from build123d import *

# Parameters (mm, degrees)
SKETCH1_R               = 5
BOSS_EXTRUDE1_DEPTH     = 35
SKETCH1_3_R             = 8
SKETCH1_3_R_2           = 5
BOSS_EXTRUDE2_DEPTH     = 2
SKETCH3_R               = 1
CUT_EXTRUDE3_DEPTH      = 9
CUT_EXTRUDE3_DEPTH_BACK = 9
FILLET1_R               = 0.5


with BuildPart() as part:
    # Sketch1 → Boss-Extrude1 (new body)
    with BuildSketch(Plane.XY):
        Circle(SKETCH1_R)
    extrude(amount=BOSS_EXTRUDE1_DEPTH)

    # Sketch1<3> → Boss-Extrude2 (add)
    with BuildSketch(Plane.XY):
        Circle(SKETCH1_3_R)
        Circle(SKETCH1_3_R_2, mode=Mode.SUBTRACT)
    extrude(amount=BOSS_EXTRUDE2_DEPTH)

    # Sketch3 → Cut-Extrude3 (cut, two sides)
    with BuildSketch(Plane(origin=(0, 0, 0), x_dir=(0, 0, -1), z_dir=(1, 0, 0))) as cut_extrude3_sk:
        with Locations((-30, 0)):
            Circle(SKETCH3_R)
    extrude(amount=CUT_EXTRUDE3_DEPTH, mode=Mode.SUBTRACT)
    extrude(cut_extrude3_sk.sketch, amount=-CUT_EXTRUDE3_DEPTH_BACK, mode=Mode.SUBTRACT)

    # Fillet1
    fillet1_edges = [part.edges().sort_by_distance(p)[0] for p in [
        (-5, 0, 35),
    ]]
    fillet(fillet1_edges, radius=FILLET1_R)


solid = part.part
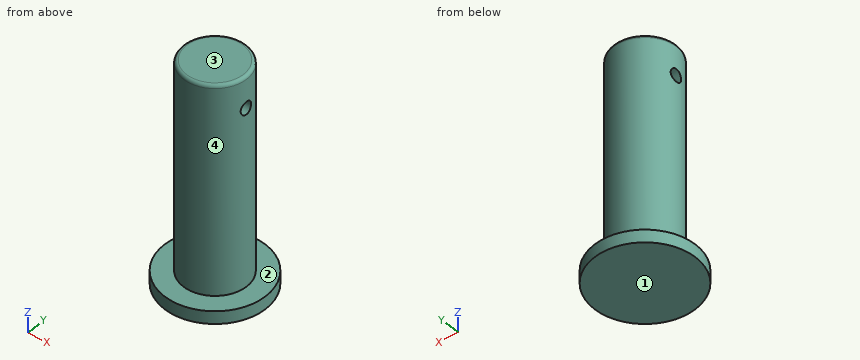
Work out the finished part from the listing and answer in its coordinate system (mm). Face numbers are marked on the shaded views. A direction names the side the tool comes from. Give positions to 0.01 mm unless a question says otherwise; leave off trailing zeros. Order: outer loops, then holes, each group sorted by start corner. A loop starts at its lowest first (then second) coordinate and runs counter-clockwise, first axis right, second up. Notation, with made-up numbers: (23, 89.25) - (52, 89.25) arc R26 ccw to (52, 110.25) - close; hole circle Ø3 at (87.25, 22.25). An arc over 180 degrees is marked (long way). Answer as CSV lines item,"result". Start each with the question number.
Q1. The part is cut by section D-D (x = 6.75). Write down the section's boundary in (y, z).
Q2. The part is cut by section C-C (z = 30). Write down the section's boundary in (x, y), then the cut area to 3 significant figures.
Q3. The part is cut by section A-A (y = 0). Write down the section's boundary in (x, z).
Q4. Given pin 1 Ø5 at (x, y) = (-4.5, -1) entering from +Z; pin 2 Ø3 at (y, z) = (0, 30) entering from -X; pin 3 Ø6 at (x, z) = (-5, 20.5) entering from -Y; pin 4 Ø8 at (x, z) = (5.5, 21) entering from -Y, each flat-ended and moving along its own axis, determine where each tip first touches the part or whether it passes through.
Q5. The mould has two halves that part along X. Classify the marked faces 3 and 4: +X half, -X half, draft (parallel to the pull), parting line (faces both ways), or undercut.
Q6. Find the intervals of material crossed by L1, parallel to Z at x = 2.05, y = 0; L2, parallel to Z at x = -0.75, y = 7.25; L3, parallel to Y at x = -3.15, z = 30, in increasing order. Write a range as [from, to].
Q7. The part is cut by section B-B (z = 17). Write down the section's boundary in (x, y).
Q8. For the marked faces 1 and 2, determine the directions among +Z, -Z, +X, -X, +Y, -Y from which every point of the face is accessible in a straight line to the end or side of a thin tool.
Check result:
1,outline,"(-4.29, 0) - (4.29, 0) - (4.29, 2) - (-4.29, 2) - close"
2,outline,"(-4.9, -1) arc R5 ccw to (4.9, -1) - close; (-4.9, 1) - (4.9, 1) arc R5 ccw to start"
2,area,"58.7 mm²"
3,outline,"(-8, 0) - (8, 0) - (8, 2) - (5, 2) - (5, 29) - (-5, 29) - (-5, 2) - (-8, 2) - close; (-5, 31) - (5, 31) - (5, 34.5) arc R0.5 ccw to (4.5, 35) - (-4.5, 35) arc R0.5 ccw to (-5, 34.5) - close"
4,pin 1,"stops at z = 35"
4,pin 2,"stops at x = -5"
4,pin 3,"stops at y = -4.58"
4,pin 4,"stops at y = -4.77"
5,face 3,"draft"
5,face 4,"parting line"
6,L1,"z = [0, 29], [31, 35]"
6,L2,"z = [0, 2]"
6,L3,"y = [-3.88, -1], [1, 3.88]"
7,outline,"circle Ø10 at (0, 0)"
8,face 1,"-Z, +X, -X, +Y, -Y"
8,face 2,"+Z"
